The model under review builds one solid part; all positions refer to its coordinate system, in mm. Round coordinates to 2 decimals unless told otherwise and drop trailing zeros. Write each loop counter-clockwise with the first axis right and the second up, starting at its lowest first coordinate (ties: lowest second). Pieces come first, ordered by that corner, then holes. Notation, with made-up numbers: (-1, -1.5) -> (15, -1.5) arc R16 ccw to (15, 15.5) -> close; hole circle Ø6 at (75, 27). An arc over 180 degrees is marked (long way). Return JSON: item names as keys, results as strings. Group by question number.
1. Take a section at C-C, the plane y = 74.9. Write out the cut boundary in (x, z), then the cut area to 3 significant figures.
2. Take a section at B-B, the plane z = 0.45. Write out the cut boundary in (x, y), then the cut area to 3 significant figures.
3. Clearance check with flat-ended pins moving along their axes: P1, Ø3, axis at x = -55.4, y = 74.9, coming from the -Z side; P2, Ø4, axis at x = 55.4, y = 47.16, coming from the -Z side. State where each tip first meets the part, or that it passes through.
4. Take a section at D-D, the plane x = 26.5. Write out the cut boundary in (y, z), then the cut area to 3 significant figures.
5. Take a section at A-A, the plane y = 5.1. Write out the cut boundary in (x, z).
6. For line 1 along X through (y, z) = (5.1, 0.75); line 2 along Y through (x, z) = (-55.4, 0.4); line 3 along Y through (x, z) = (12, 2.4), list the stretches that pass through material, from the lowest coordinate up. Write a range as from..to.
from build123d import *

# Parameters (mm, degrees)
EXTRUDE_1_DEPTH            = 3
HOLE_WIZARD_M31_AT_2_COUNT = 2
HOLE_WIZARD_M31_AT_2_PITCH = 69.828647416
HOLE_WIZARD_M31_AT_3_COUNT = 2
HOLE_WIZARD_M31_AT_3_PITCH = 114.220491135
HOLE_WIZARD_M31_AT_4_COUNT = 2
HOLE_WIZARD_M31_AT_4_PITCH = 132.649462871


with BuildPart() as part:
    # Эскиз1 → Бобышка-Вытянуть1 (new body)
    with BuildSketch(Plane.XY):
        Polygon((-19.924322584, 80), (62.5, 50), (62.5, 0), (-62.5, 0), (-62.5, 80), align=None)
    extrude(amount=EXTRUDE_1_DEPTH)

    # Эскиз5 → Зенковка для винта с потайной головкой M31 (revolve, cut)
    with BuildSketch(Plane(origin=(-55.4, 74.9, 3), x_dir=(0, -1, 0), z_dir=(1, 0, 0))):
        Polygon((0, 0), (0, 3), (1.7, 3), (1.7, 1.45), (3.15, 0), align=None)
    hole_wizard_m31 = revolve(axis=Axis((-55.4, 74.9, 9.35), (0, 0, -1)), mode=Mode.SUBTRACT)

    # Зенковка для винта с потайной головкой M31 at 2: Зенковка для винта с потайной головкой M31 ×2
    with Locations(*[Vector(-0.02864154002689579, -0.9995897469386568, 0) * (i * HOLE_WIZARD_M31_AT_2_PITCH) for i in range(1, HOLE_WIZARD_M31_AT_2_COUNT)]):
        add(hole_wizard_m31, mode=Mode.SUBTRACT)

    # Зенковка для винта с потайной головкой M31 at 3: Зенковка для винта с потайной головкой M31 ×2
    with Locations(*[Vector(0.9700536120909078, -0.24289090075460365, 0) * (i * HOLE_WIZARD_M31_AT_3_PITCH) for i in range(1, HOLE_WIZARD_M31_AT_3_COUNT)]):
        add(hole_wizard_m31, mode=Mode.SUBTRACT)

    # Зенковка для винта с потайной головкой M31 at 4: Зенковка для винта с потайной головкой M31 ×2
    with Locations(*[Vector(0.8503615284864274, -0.5261988890811409, 0) * (i * HOLE_WIZARD_M31_AT_4_PITCH) for i in range(1, HOLE_WIZARD_M31_AT_4_COUNT)]):
        add(hole_wizard_m31, mode=Mode.SUBTRACT)


solid = part.part
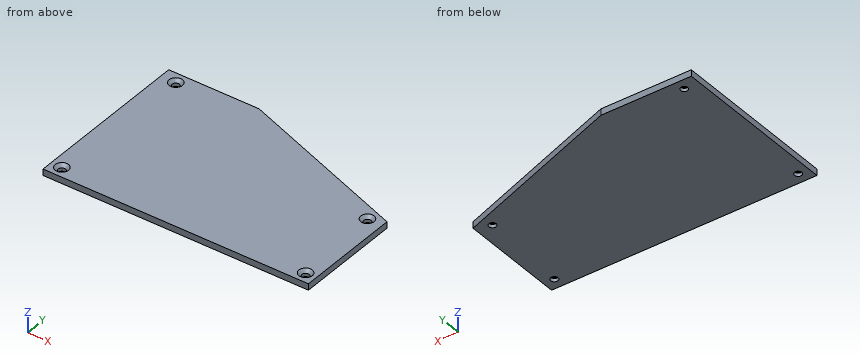
Output:
{
 "1": {"outline": "(-62.5, 0) -> (-57.1, 0) -> (-57.1, 1.55) -> (-58.55, 3) -> (-62.5, 3) -> close; (-53.7, 0) -> (-5.91, 0) -> (-5.91, 3) -> (-52.25, 3) -> (-53.7, 1.55) -> close", "area": "157 mm^2"},
 "2": {"outline": "(-62.5, 0) -> (62.5, 0) -> (62.5, 50) -> (-19.92, 80) -> (-62.5, 80) -> close; hole circle Ø3.4 at (-57.4, 5.1); hole circle Ø3.4 at (-55.4, 74.9); hole circle Ø3.4 at (55.4, 47.16); hole circle Ø3.4 at (57.4, 5.1)", "area": "8,730 mm^2"},
 "3": {"P1": "passes through", "P2": "stops at z = 0"},
 "4": {"outline": "(0, 0) -> (63.1, 0) -> (63.1, 3) -> (0, 3) -> close", "area": "189 mm^2"},
 "5": {"outline": "(-62.5, 0) -> (-59.1, 0) -> (-59.1, 1.55) -> (-60.55, 3) -> (-62.5, 3) -> close; (-55.7, 0) -> (55.7, 0) -> (55.7, 1.55) -> (54.25, 3) -> (-54.25, 3) -> (-55.7, 1.55) -> close; (59.1, 0) -> (62.5, 0) -> (62.5, 3) -> (60.55, 3) -> (59.1, 1.55) -> close"},
 "6": {"line 1": "x = -62.5..-59.1, -55.7..55.7, 59.1..62.5", "line 2": "y = 0..73.2, 76.6..80", "line 3": "y = 0..68.38"}
}
